The listing builds one solid part. Answer for the finished solid, in the listing's coordinates (mm). Face numbers are marked on the shaded views. A direction names the side the tool comes from. Coordinates: 2 decimals unless noted, no trailing zeros. Write each loop counter-clockwise with the first axis right and the second up, starting at its lowest first coordinate (ties: lowest second). Pieces come first, ordered by that corner, then holes.
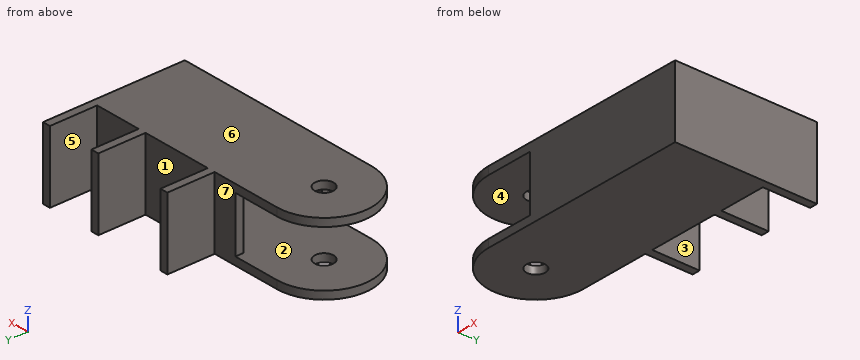
from build123d import *

# Parameters (mm, degrees)
DODANIE_WYCI_GNI_CIE1_DEPTH = 5
SZKIC2_W                    = 100
SZKIC2_H                    = 35
DODANIE_WYCI_GNI_CIE2_DEPTH = 5
SZKIC3_R                    = 6
WYTNIJ_WYCI_GNI_CIE1_DEPTH  = 110.316055545
SZKIC4_W                    = 5
SZKIC4_H                    = 30
SZKIC4_H_2                  = 90
DODANIE_WYCI_GNI_CIE3_DEPTH = 45


with BuildPart() as part:
    # Szkic1 → Dodanie-wyci_gni_cie1 (new body)
    with BuildSketch(Plane.XY):
        with BuildLine():
            Line((-65, -30), (65, -30))
            Line((65, -30), (65, 30))
            Line((65, 30), (-65, 30))
            ThreePointArc((-65, 30), (-95, 0), (-65, -30))
        make_face()
    extrude(amount=DODANIE_WYCI_GNI_CIE1_DEPTH)


with BuildPart() as body_2:
    # Lustro2: mirrored copy
    add(part.part.mirror(Plane.XY.offset(22.5)))


with BuildPart() as part_1:
    add(part.part)

    add(body_2.part)  # Dodanie-wyci_gni_cie2 merges body 2
    # Szkic2 → Dodanie-wyci_gni_cie2 (add)
    with BuildSketch(Plane(origin=(0, 30, 0), x_dir=(1, 0, 0), z_dir=(0, 1, 0))):
        with Locations((15, -22.5)):
            Rectangle(SZKIC2_W, SZKIC2_H)
    dodanie_wyci_gni_cie2 = extrude(amount=-DODANIE_WYCI_GNI_CIE2_DEPTH)

    # Lustro3: Dodanie-wyci_gni_cie2 across plane
    add(dodanie_wyci_gni_cie2.mirror(Plane.ZX))

    # Szkic3 → Wytnij-wyci_gni_cie1 (cut, through all)
    with BuildSketch(Plane.XY.offset(45)):
        with Locations((-65, 0)):
            Circle(SZKIC3_R)
    extrude(amount=-WYTNIJ_WYCI_GNI_CIE1_DEPTH, mode=Mode.SUBTRACT)

    # Szkic4 → Dodanie-wyci_gni_cie3 (add)
    with BuildSketch(Plane.XY.offset(45)):
        with Locations((32.5, 45)):
            Rectangle(SZKIC4_W, SZKIC4_H)
        with Locations((67.5, 15)):
            Rectangle(SZKIC4_W, SZKIC4_H_2)
        with Locations((-17.5, 45)):
            Rectangle(SZKIC4_W, SZKIC4_H)
    extrude(amount=-DODANIE_WYCI_GNI_CIE3_DEPTH)


solid = part_1.part
Q1. The part is cut by section B-B, the plane x = -2. Write down the section's boundary in (y, z), then the cut area to 3 significant figures.
Answers below:
outline: (-30, 0) - (30, 0) - (30, 45) - (-30, 45) - close; hole (-25, 5) - (25, 5) - (25, 40) - (-25, 40) - close
area: 950 mm2
Q2. Given pin 1 (11 mm diameter, centred on x = -65, y = 0, fed in from +Z); pin 2 (12 mm diameter, centred on y = 18, z = 9.5, fed in from -X); pin 3 (9 mm diameter, centred on y = 38, z = 27, fed in from -X); pin 4 (24 mm diameter, centred on x = 50.5, z = 11.5, fed in from +Y), each flat-ended and moving along its own axis, determine where each tip first touches the part or whether it passes through.
Answers below:
pin 1: passes through
pin 2: stops at x = -91.52
pin 3: stops at x = -20
pin 4: stops at y = 30
Q3. The part is cut by section A-A, the plane y = 34. Write down the section's boundary in (x, z).
Answers below:
outline: (-20, 0) - (-15, 0) - (-15, 45) - (-20, 45) - close; (30, 0) - (35, 0) - (35, 45) - (30, 45) - close; (65, 0) - (70, 0) - (70, 45) - (65, 45) - close
Q4. Which of the six approach directions +Z, -Z, +X, -X, +Y, -Y give full straight-line access (tool end or side, diameter ignored) to the marked faces 5, 6 and 7?
Answers below:
face 5: +Z, -Z, +Y
face 6: +Z, +X, -X, +Y, -Y
face 7: +Z, -Z, -X, +Y
Q5. Find the intervals of material crossed by probe 1 along X at (y, z) = (55, 32); probe 2 along Y at (x, z) = (-10, 27.5); probe 3 along Z at (x, y) = (57, 14), in increasing order.
Answers below:
probe 1: x = -20 to -15, 30 to 35, 65 to 70
probe 2: y = -30 to -25, 25 to 30
probe 3: z = 0 to 5, 40 to 45
Q6. Determine the mould class of the marked faces 1, 2, 3 and 4 for opening direction Y: released by +Y, released by -Y, zero draft, split by the parting line, or undercut.
Answers below:
face 1: released by +Y
face 2: undercut
face 3: zero draft
face 4: undercut
Q7. The part is cut by section C-C, the plane x = -55. Write down the section's boundary in (y, z).
Answers below:
outline: (-30, 0) - (30, 0) - (30, 5) - (-30, 5) - close; (-30, 40) - (30, 40) - (30, 45) - (-30, 45) - close
Q8. The part is cut by section D-D, the plane y = 0. Write down the section's boundary in (x, z), then the cut area to 4 significant figures.
Answers below:
outline: (-95, 0) - (-71, 0) - (-71, 5) - (-95, 5) - close; (-95, 40) - (-71, 40) - (-71, 45) - (-95, 45) - close; (-59, 0) - (70, 0) - (70, 45) - (-59, 45) - (-59, 40) - (65, 40) - (65, 5) - (-59, 5) - close
area: 1,705 mm2
